Verification items for the finished model (mm, model axes). Face numbers are marked on the shaded views. Coordinates: 2 decimals unless noted, no trailing zeros. Order: outer loops, then holes, each group sorted by start corner. A loop starts at its lowest first (then second) coordinate and runs counter-clockwise, first axis right, second up.
Q1. Thickness scan on line 1 (Y direction, x = -51.5, z = 6.5); line 2 (X direction, y = -481.5, z = 25.5); line 3 (X direction, y = 12, z = -43.5). Record the ranges inside material, lowest first.
Q2. Cross-section at B-B, the plane x = -17. Record the boundary of the cut face in (y, z), and give its area (3 significant figures).
Q3. Draft check along Y on the marked faces 1, 2, 3 and 4. Enter one of: pulls with the +Y half, pulls with the -Y half, needs draft (parallel to the pull), parting line crosses it, or undercut.
Q4. Depth check by flat-ended pin: P1, Ø6, axis at y = -55.5, z = -2.5, coming from the -X side; P2, Ø1.5, axis at y = -56.5, z = 3, coming from the -X side; P3, Ø4, axis at x = 57.5, z = -37.5, coming from the -Y side. Enter the tip coordinate at first touch or a pass-through.
Q5. Cross-section at A-A, the plane z = -37. Record the boundary of the cut face in (x, y), and give its area (3 significant figures).
Q6. Cross-section at C-C, the plane y = -61. Record the boundary of the cut face in (x, z), and give its area (3 significant figures).
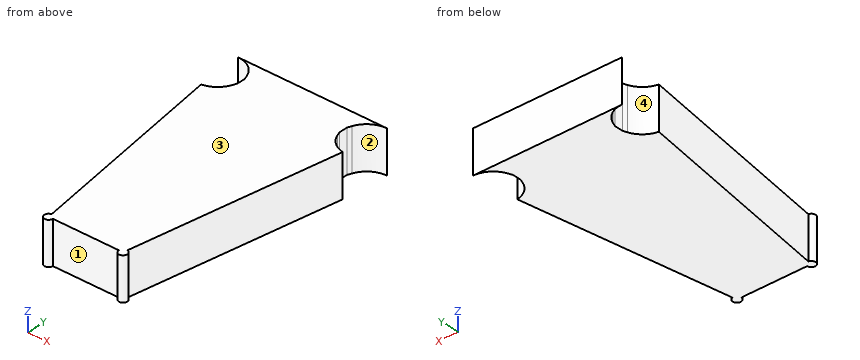
Autodesk Inventor part; units mm, degrees
ref_plane "YZ Plane" through (0, 0, 0) normal (1, 0, 0) x (0, 1, 0)
ref_plane "XZ Plane" through (0, 0, 0) normal (0, 1, 0) x (-1, 0, 0)
ref_plane "XY Plane" through (0, 0, 0) normal (0, 0, 1) x (1, 0, 0)
sketch "Эскиз1" plane through (0, 0, 0) normal (0, 0, 1) x (1, 0, 0)
  line L0 (-175, 0) -> (175, 0)
  line L1 (0, 0) -> (0, -465)
  line L2 (0, -465) -> (-87.5, -555)
  line L3 (-87.5, -555) -> (87.5, -555)
  line L4 (87.5, -555) -> (0, -465)
  circle A0 centre (175, 0) radius 55
  circle A1 centre (-175, 0) radius 55
  circle A2 centre (87.5, -555) radius 70
  circle A3 centre (-87.5, -555) radius 70
  line L5 (175, 0) -> (87.5, -555)
  line L6 (-175, 0) -> (-87.5, -555)
  line L7 (175, 55) -> (-175, 55)
  line L8 (87.5, -625) -> (-87.5, -625)
  line L9 (-120, 10) -> (-120, -10)
  line L10 (120, 10) -> (120, -10)
  line L11 (-120, 10) -> (-123.52, 19.36)
  line L12 (-120, -10) -> (-123.52, -19.36)
  line L13 (120, 10) -> (123.52, 19.36)
  line L14 (120, -10) -> (123.52, -19.36)
  circle A4 centre (87.5, -555) radius 10
  circle A5 centre (-87.5, -555) radius 10
  point P0 (0, -555)
  point P1 (166.4346, -54.3289)
  point P2 (-166.4346, -54.3289)
  point P3 (-98.4014, -485.8541)
  point P4 (98.4014, -485.8541)
  point P5 (120, 0)
  point P6 (-120, 0)
  point P7 (-38.7045, -504.8104)
  point P8 (38.7045, -504.8104)
  point P9 (89.0573, -545.122)
  point P10 (-89.0573, -545.122)
  point P11 (-77.5, -555)
  point P12 (77.5, -555)
  dimension "d10" = 140
  dimension "d11" = 140
  dimension "d4" = 90
  dimension "d5" = 175
  dimension "d6" = 350
  dimension "d7" = 110
  dimension "d8" = 110
  dimension "d9" = 465
  dimension "d14" = 20
  dimension "d15" = 20
  dimension "d16" = 20
  dimension "d17" = 20
extrude "Выдавливание1" add sketch "Эскиз1" along normal mid plane 100 contours L9 L11 A1 L7 A0 L13 L10 L0 | L0 L1 L2 A3 L6 A1 L12 L9 | L0 L10 L14 A0 L5 A2 L4 L1 | A3 L2 A5 L6 | L4 A2 L3 A3 L2 | A3 L3 A5 L2 | A5 L2 L6 | L6 L3 A5 | A2 L5 A4 L4 | L4 A4 L3 A2 | A5 L3 L2 | A4 L5 L4 | L4 L3 A4 | L5 A4 L3
equation "\"d10\" = hip_diam"
equation "\"d11\" = d10"
equation "\"d4\" = hip_joint_hight"
equation "\"d5\" = hip_joint_width"
equation "\"d6\" = clavicular_width"
equation "\"d7\" = shoulder_radius"
equation "\"d8\" = d7"
properties part number "ч ASY human dummy 01"
Check values:
1. line 1: y = -555 to 55
1. line 2: x = -99.09 to 99.09
1. line 3: x = -120.75 to 120.75
2. outline: (-555, -50) - (55, -50) - (55, 50) - (-555, 50) - close
2. area: 61,000 mm2
3. face 1: pulls with the -Y half
3. face 2: undercut
3. face 3: needs draft
3. face 4: undercut
4. P1: stops at x = -166.43
4. P2: stops at x = -166.21
4. P3: stops at y = -555
5. outline: (-175, 55) arc R55 cw to (-123.52, 19.36) - (-120, 10) - (-120, -10) - (-123.52, -19.36) arc R55 cw to (-166.43, -54.33) - (-89.06, -545.12) arc R10 ccw (long way) to (-77.5, -555) - (77.5, -555) arc R10 ccw (long way) to (89.06, -545.12) - (166.43, -54.33) arc R55 cw to (123.52, -19.36) - (120, -10) - (120, 10) - (123.52, 19.36) arc R55 cw to (175, 55) - close
5. area: 156,000 mm2
6. outline: (-165.38, -50) - (165.38, -50) - (165.38, 50) - (-165.38, 50) - close
6. area: 33,100 mm2
